Here's how the part is built. I have some questions about the finished solid (model axes, mm). A direction names the side the tool comes from. Round coordinates to 2 decimals unless told otherwise and drop trailing zeros. Write each loop counter-clockwise with the first axis right and the second up, starting at its lowest first coordinate (ties: lowest second). Pieces come first, ordered by that corner, then holes. Notation, with made-up numbers: (69.25, 81.5) - (96.25, 81.5) arc R16 ccw to (96.25, 99.5) - close; hole circle Ø10 at (-4, 8.25). An arc over 180 degrees is marked (long way). Return JSON: item names as keys, results as strings. Group by question number.
```python
from build123d import *

# Parameters (mm, degrees)
BOSS_EXTRUDE1_DEPTH     = 3.175
FILLET1_R               = 20
SKETCH2_R               = 2.25
CUT_EXTRUDE1_DEPTH      = 164.037303514
CUT_EXTRUDE2_DEPTH      = 164.037303514
CUT_EXTRUDE2_DEPTH_BACK = 164.037303514
SKETCH3_R               = 1.25
CUT_EXTRUDE3_DEPTH      = 164.037303514
CUT_EXTRUDE3_DEPTH_BACK = 164.037303514
FILLET2_R               = 2


with BuildPart() as part:
    # Sketch1 → Boss-Extrude1 (new, symmetric)
    with BuildSketch(Plane.XY):
        with BuildLine():
            Line((43.566419732, -16.254755357), (100, 135))
            Line((100, 135), (-100, 135))
            Line((-100, 135), (-43.566419732, -16.254755357))
            ThreePointArc((-43.566419732, -16.254755357), (0, -46.5), (43.566419732, -16.254755357))
        make_face()
    extrude(amount=BOSS_EXTRUDE1_DEPTH, both=True)

    # Fillet1
    fillet1_edges = [part.edges().sort_by_distance(p)[0] for p in [
        (-100, 135, 0),
        (100, 135, 0),
    ]]
    fillet(fillet1_edges, radius=FILLET1_R)

    # Sketch2 → Cut-Extrude1 (cut, through all)
    with BuildSketch(Plane(origin=(0, 0, -3.175), x_dir=(-1, 0, 0), z_dir=(0, 0, -1))):
        with Locations((-71.191226755, 115)):
            Circle(SKETCH2_R)
        with Locations((71.191226755, 115)):
            Circle(SKETCH2_R)
        with Locations((0, 90.999999998)):
            Circle(SKETCH2_R)
    extrude(amount=-CUT_EXTRUDE1_DEPTH, mode=Mode.SUBTRACT)

    # Sketch3 → Cut-Extrude2 (cut, two sides: drawn at the far end of the back side and taken through both)
    with BuildSketch(Plane(origin=(0, 0, -3.175), x_dir=(-1, 0, 0), z_dir=(0, 0, -1)).offset(-CUT_EXTRUDE2_DEPTH_BACK)):
        with Locations((17.440159599, -16.121517706)):
            Circle(SKETCH3_R)
        with Locations((22.282044228, -8.220280106)):
            Circle(SKETCH3_R)
        with Locations((9.943168767, -21.568400378)):
            Circle(SKETCH3_R)
        with Locations((0.932420624, -23.731689611)):
            Circle(SKETCH3_R)
        with Locations((-8.220280106, -22.282044228)):
            Circle(SKETCH3_R)
        with Locations((-16.121517706, -17.440159599)):
            Circle(SKETCH3_R)
        with Locations((-21.568400378, -9.943168767)):
            Circle(SKETCH3_R)
        with Locations((-23.731689611, -0.932420624)):
            Circle(SKETCH3_R)
        with Locations((-22.282044228, 8.220280106)):
            Circle(SKETCH3_R)
        with Locations((-17.440159599, 16.121517706)):
            Circle(SKETCH3_R)
        with Locations((-9.943168767, 21.568400378)):
            Circle(SKETCH3_R)
        with Locations((-0.932420624, 23.731689611)):
            Circle(SKETCH3_R)
        with Locations((8.220280106, 22.282044228)):
            Circle(SKETCH3_R)
        with Locations((16.121517706, 17.440159599)):
            Circle(SKETCH3_R)
        with Locations((21.568400378, 9.943168767)):
            Circle(SKETCH3_R)
        with Locations((23.731689611, 0.932420624)):
            Circle(SKETCH3_R)
    extrude(amount=CUT_EXTRUDE2_DEPTH + CUT_EXTRUDE2_DEPTH_BACK, mode=Mode.SUBTRACT)

    # Sketch4 → Cut-Extrude3 (cut, two sides: drawn at the far end of the back side and taken through both)
    with BuildSketch(Plane.XY.offset(3.175).offset(-CUT_EXTRUDE3_DEPTH_BACK)):
        Polygon((-63.696742607, 102.893653244), (-50.607894628, 56.486565879), (-14.905780513, 24.078314663), (-27.994628493, 70.485402028), align=None)
        Polygon((63.696742607, 102.893653244), (50.607894628, 56.486565879), (14.905780513, 24.078314663), (27.994628493, 70.485402028), align=None)
        Polygon((0, 85.183808507), (-9.976320033, 56.751243307), (0, 28.318678107), (9.976320033, 56.751243307), align=None)
        Polygon((-56.952865739, 115), (0, 127.073716961), (56.952865739, 115), (0, 102.926283039), align=None)
        Polygon((-46.602642472, 42.285767842), (-45.512737624, 19.397766035), (-34.482528345, -0.686630956), (-35.572433193, 22.20137085), align=None)
        Polygon((46.602642472, 42.285767842), (35.572433193, 22.20137085), (34.482528345, -0.686630956), (45.512737624, 19.397766035), align=None)
    extrude(amount=CUT_EXTRUDE3_DEPTH + CUT_EXTRUDE3_DEPTH_BACK, mode=Mode.SUBTRACT)

    # Fillet2
    fillet2_edges = [part.edges().sort_by_distance(p)[0] for p in [
        (-46.602642472, 42.285767842, 0),
        (-35.572433193, 22.20137085, 0),
        (-34.482528345, -0.686630956, 0),
        (-45.512737624, 19.397766035, 0),
        (0, 85.183808507, 0),
        (9.976320033, 56.751243307, 0),
        (0, 28.318678107, 0),
        (-9.976320033, 56.751243307, 0),
        (0, 102.926283039, 0),
        (-56.952865739, 115, 0),
        (0, 127.073716961, 0),
        (56.952865739, 115, 0),
        (27.994628493, 70.485402028, 0),
        (63.696742607, 102.893653244, 0),
        (50.607894628, 56.486565879, 0),
        (14.905780513, 24.078314663, 0),
        (46.602642472, 42.285767842, 0),
        (45.512737624, 19.397766035, 0),
        (34.482528345, -0.686630956, 0),
        (35.572433193, 22.20137085, 0),
        (-63.696742607, 102.893653244, 0),
        (-27.994628493, 70.485402028, 0),
        (-14.905780513, 24.078314663, 0),
        (-50.607894628, 56.486565879, 0),
    ]]
    fillet(fillet2_edges, radius=FILLET2_R)


solid = part.part
```
1) For faces 4 (the flat face through (1, 135, 0)), 5 (the flat face through (-43.27, 84.35, -0.04)), which set-ups out of +Z, -Z, +X, -X, +Y, -Y let a thin tool reach every point of the face, with its end or its side?
2) Imagine slicing it at B-B (y = 91). Please give me the cut outline in (x, z) (3 decimals).
3) Imagine slicing it at D-D (x = 79). Please give me the cut outline in (y, z) (3 decimals), plus the area to 3 significant figures.
4) Imagine slicing it at A-A (y = 122.5). Please give me the cut outline in (x, z) (3 decimals), plus the area to 3 significant figures.
5) Imagine slicing it at C-C (z = 2). Give the number of separate pieces and of enclosed holes in the cut face, plus the area to 3 significant figures.
6) I need wall thicknesses on line 1 along Y through (x, z) = (36, 2.5); line 2 along X through (y, z) = (63.5, -0.5); line 3 along Y through (x, z) = (-16, -1). Which ranges of each line are inside material? Lowest first, please.
7) Will these pins go through, and if not, where does the flat tip stop? pin 1 Ø1.5 at (y, z) = (78, 1) entering from -X; pin 2 Ø2 at (x, y) = (17.44, 16.12) entering from +Z.
8) If we mould it in two halves opening along X, with no side actions, what happens to faces 1 (the cylindrical face through (-0.79, -46.493, 0.044)), 2 (the flat face through (66.423, 45.007, 0.044)), 3 (the flat face through (24.4, 108.1, 0))? For each: released by +X, released by -X, zero draft, split by the parting line, or undercut.
Results found:
{
 "1": {"face 4": "+Z, -Z, +X, -X, +Y", "face 5": "+Z, -Z"},
 "2": {"outline": "(-83.583, -3.175) - (-60.342, -3.175) - (-60.342, 3.175) - (-83.583, 3.175) - close; (-50.594, -3.175) - (-2.25, -3.175) - (-2.25, 3.175) - (-50.594, 3.175) - close; (2.25, -3.175) - (50.594, -3.175) - (50.594, 3.175) - (2.25, 3.175) - close; (60.342, -3.175) - (83.583, -3.175) - (83.583, 3.175) - (60.342, 3.175) - close"},
 "3": {"outline": "(78.715, -3.175) - (133.413, -3.175) - (133.413, 3.175) - (78.715, 3.175) - close", "area": "347 mm²"},
 "4": {"outline": "(-89.732, -3.175) - (-21.575, -3.175) - (-21.575, 3.175) - (-89.732, 3.175) - close; (21.575, -3.175) - (89.732, -3.175) - (89.732, 3.175) - (21.575, 3.175) - close", "area": "866 mm²"},
 "5": {"separate pieces": "1", "enclosed holes": "25", "area": "18,400 mm²"},
 "6": {"line 1": "y = -29.43 to 6.06, 22.98 to 43.23, 77.75 to 110.56, 119.44 to 135", "line 2": "x = -73.32 to -52.59, -26.02 to -7.61, 7.61 to 26.02, 52.59 to 73.32", "line 3": "y = -43.66 to 16.2, 18.68 to 106.32, 123.68 to 135"},
 "7": {"pin 1": "stops at x = -79.01", "pin 2": "passes through"},
 "8": {"face 1": "split by the parting line", "face 2": "released by +X", "face 3": "undercut"}
}
